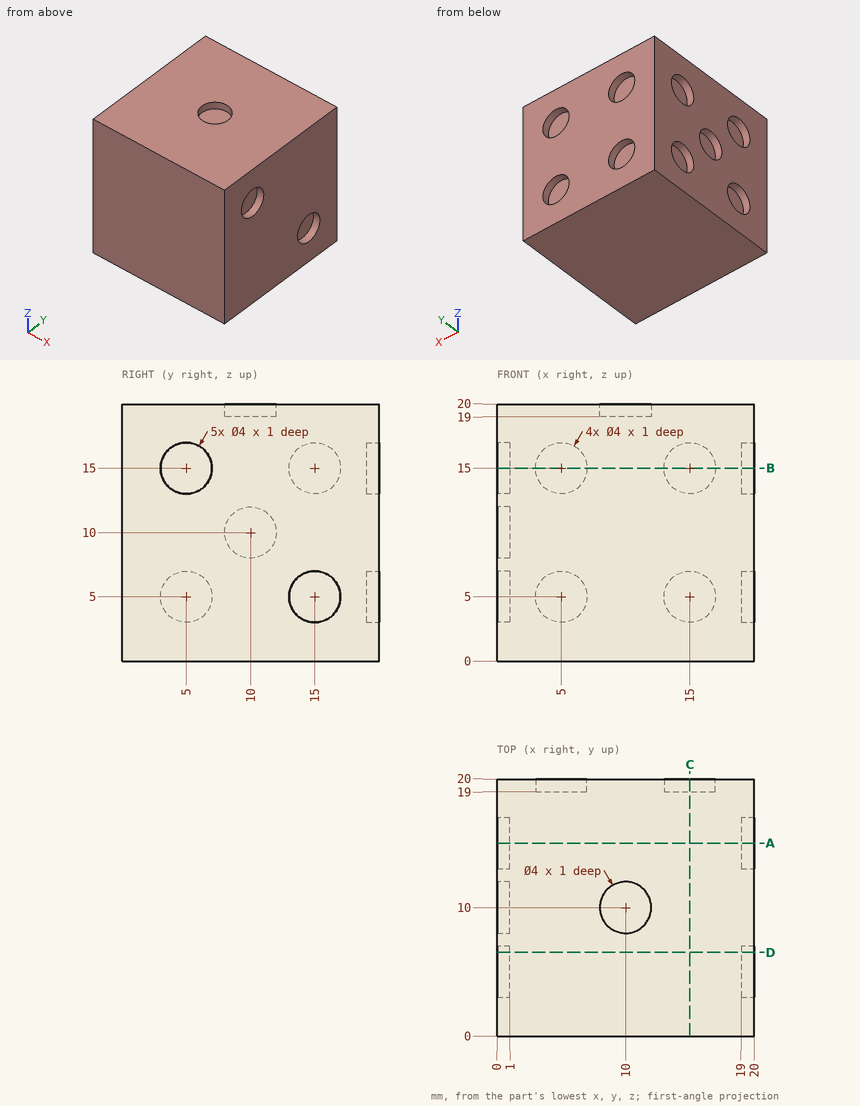
The drawing under review shows one solid part. Ordinate dimensions are in mm from its lowest x, y, z. Give positions to 0.01 mm unless a question says otherwise; leave off trailing zeros. Order: outer loops, then holes, each group sorted by start corner. A loop starts at its lowest first (then second) coordinate and runs counter-clockwise, first axis right, second up. Notation, with made-up numbers: (9.5, 37.25) -> (60.5, 37.25) arc R30 ccw to (60.5, 71.25) -> close; hole circle Ø6 at (14, 2). An arc over 180 degrees is marked (long way). Write item = value, one per line. Start each with the question number.
(1) We need section A-A on y = 15. Write out the cut boundary in (x, z).
(2) For pin 1 (1.2 mm diameter, centred on y = 5.5, z = 5, fed in from -X); pin 2 (5 mm diameter, centred on x = 15, z = 15, fed in from -Y); pin 3 (2.5 mm diameter, centred on x = 5, z = 15, fed in from +Y); pin 4 (2.5 mm diameter, centred on x = 10, y = 10, fed in from +Z), all flat-tipped, find the tip position at first contact; note any pin that passes through.
(3) We need section B-B on z = 15. Write out the cut boundary in (x, y).
(4) We need section C-C on x = 15. Write out the cut boundary in (y, z).
(5) To check wall thickness, follow line 1 along Y through (x, z) = (15, 6.5). State the ranges of the line that lie inside material, in increasing order.
(6) We need section D-D on y = 6.5. Write out the cut boundary in (x, z), plus the area to 3 significant figures.
Numbers:
q1.outline = (0, 0) -> (20, 0) -> (20, 3) -> (19, 3) -> (19, 7) -> (20, 7) -> (20, 20) -> (0, 20) -> (0, 17) -> (1, 17) -> (1, 13) -> (0, 13) -> (0, 7) -> (1, 7) -> (1, 3) -> (0, 3) -> close
q2.pin_1 = 1
q2.pin_2 = 0
q2.pin_3 = 19
q2.pin_4 = 19
q3.outline = (0, 0) -> (20, 0) -> (20, 3) -> (19, 3) -> (19, 7) -> (20, 7) -> (20, 20) -> (17, 20) -> (17, 19) -> (13, 19) -> (13, 20) -> (7, 20) -> (7, 19) -> (3, 19) -> (3, 20) -> (0, 20) -> (0, 17) -> (1, 17) -> (1, 13) -> (0, 13) -> (0, 7) -> (1, 7) -> (1, 3) -> (0, 3) -> close
q4.outline = (0, 0) -> (20, 0) -> (20, 3) -> (19, 3) -> (19, 7) -> (20, 7) -> (20, 13) -> (19, 13) -> (19, 17) -> (20, 17) -> (20, 20) -> (0, 20) -> close
q5.line_1 = 0 to 19
q6.outline = (0, 0) -> (20, 0) -> (20, 13.68) -> (19, 13.68) -> (19, 16.32) -> (20, 16.32) -> (20, 20) -> (0, 20) -> (0, 16.32) -> (1, 16.32) -> (1, 13.68) -> (0, 13.68) -> (0, 6.32) -> (1, 6.32) -> (1, 3.68) -> (0, 3.68) -> close
q6.area = 392 mm^2
